Verification items for the finished model (mm, model axes). A direction names the side the tool comes from. Coordinates: 2 decimals unless noted, no trailing zeros. Loops run counter-clockwise (first coordinate to the right, second up) from the corner with the lowest first, then second, coordinate; pieces in that order, holes last. Notation, with made-up numbers: (-25, -25.75) - (10, -25.75) arc R12 ccw to (10, -9.75) - close; hole circle Ø6 at (9.25, 51.5). An arc over 180 degrees is marked (long way). Answer as CSV lines item,"result". Start each with the question number.
1. Cross-section at C-C (z = -14). Enter the section's corners in (x, y).
2. Material ranges on line 1 (X direction, y = -0.5, z = -17.5); line 2 (Y direction, x = -0.25, z = 26); line 3 (Z direction, x = -7.25, y = -0.25), recorded low to high. Write a range as [from, to].
3. Release check for a two-part mould opening along X. For faces 5 (the flat face through (3, 0, -30)), 6 (the cylindrical face through (-2.17, -9.76, -14.85)), 7 (the flat face through (2.5, 0, -23)) record: pulls with the +X half, pulls with the -X half, needs draft (parallel to the pull), parting line crosses it, or undercut.
4. Gauge pin test, flat ends, axial feed: P1, Ø1.5, axis at x = -1, z = -25, coming from the +Y side; P2, Ø4, axis at x = -1, z = 0, coming from the +Y side; P3, Ø3, axis at y = -4.5, z = 2.5, coming from the +X side. Record the tip position at first contact, or that the pin passes through.
5. Set-up check for faces 1 (the flat face through (2.5, 0, 23)), 2 (the flat face through (0, 1.9, -23)), 3 (the cylindrical face through (-2.17, -9.76, 14.85)), 4 (the conical face through (5.9, 1.9, 0.2)): record each of +Z, -Z, +X, -X, +Y, -Y from which the full face is reachable in a straight line by a thin tool's end or side.
6. Cross-section at A-A (y = 0). Enter the section's corners in (x, z).
7. Cross-section at B-B (x = 0). Enter the section's corners in (y, z).
```python
from build123d import *

# Parameters (mm, degrees)
F0_R     = 10
F1_DEPTH = 30
F2_W     = 5
F2_H     = 3.8
F3_DEPTH = 15
F4_R     = 4
F5_SIZE  = 4


with BuildPart() as f1:
    # F0 (on Top) → F1 (new body)
    with BuildSketch(Plane.XY):
        Circle(F0_R)
    extrude(amount=F1_DEPTH)

    # F2 (on face) → F3 (cut)
    with BuildSketch(Plane.XY.offset(30)):
        Rectangle(F2_W, F2_H)
    extrude(amount=-F3_DEPTH, mode=Mode.SUBTRACT)

    # F4
    f4_edges = [f1.edges().sort_by_distance(p)[0] for p in [
        (-10, 0, 30),
    ]]
    fillet(f4_edges, radius=F4_R)

    # F5
    f5_edges = [f1.edges().sort_by_distance(p)[0] for p in [
        (-10, 0, 0),
    ]]
    chamfer(f5_edges, length=F5_SIZE)

    # F6: F1 across face


with BuildPart() as f1_1:
    add(f1.part)
    add(f1.part.mirror(Plane(origin=(0, 0, 0), x_dir=(1, 0, 0), z_dir=(0, 0, -1))))


solid = f1_1.part
```
Values follow:
1,outline,"circle Ø20 at (0, 0)"
2,line 1,"x = [-9.99, -2.5], [2.5, 9.99]"
2,line 2,"y = [-10, -1.9], [1.9, 10]"
2,line 3,"z = [-29.8, -1.25], [1.25, 29.8]"
3,face 5,"needs draft"
3,face 6,"parting line crosses it"
3,face 7,"undercut"
4,P1,"stops at y = 10"
4,P2,"stops at y = 7.95"
4,P3,"stops at x = 9.07"
5,face 1,"+Z"
5,face 2,"-Z"
5,face 3,"+Z, -Z"
5,face 4,"none"
6,outline,"(-10, -26) arc R4 ccw to (-6, -30) - (-2.5, -30) - (-2.5, -15) - (2.5, -15) - (2.5, -30) - (6, -30) arc R4 ccw to (10, -26) - (10, -4) - (6, 0) - (10, 4) - (10, 26) arc R4 ccw to (6, 30) - (2.5, 30) - (2.5, 15) - (-2.5, 15) - (-2.5, 30) - (-6, 30) arc R4 ccw to (-10, 26) - (-10, 4) - (-6, 0) - (-10, -4) - close"
7,outline,"(-10, -26) arc R4 ccw to (-6, -30) - (-1.9, -30) - (-1.9, -15) - (1.9, -15) - (1.9, -30) - (6, -30) arc R4 ccw to (10, -26) - (10, -4) - (6, 0) - (10, 4) - (10, 26) arc R4 ccw to (6, 30) - (1.9, 30) - (1.9, 15) - (-1.9, 15) - (-1.9, 30) - (-6, 30) arc R4 ccw to (-10, 26) - (-10, 4) - (-6, 0) - (-10, -4) - close"
